from build123d import *

# Parameters (mm, degrees)
SKETCH2_OUTSIDE_W  = 26.862
SKETCH2_OUTSIDE_H  = 26.862
CUT_EXTRUDE1_DEPTH = 10
CHAMFER1_SIZE      = 0.5


with BuildPart() as part:
    # Sketch1 → Revolve1 (revolve)
    with BuildSketch(Plane(origin=(0, 0, 0), x_dir=(0, 0, -1), z_dir=(1, 0, 0)), mode=Mode.PRIVATE) as revolve1_sk:
        Polygon((0, 3.45), (0, 8.205420274), (0.373676511, 9.6), (2.426323489, 9.6), (2.8, 8.205420274), (2.8, 4.7), (4.2, 4.7), (4.2, 5.4), (7.5, 5.4), (8, 4.9), (8, 3.45), align=None)
    revolve(revolve1_sk.sketch.rotate(Axis((0, 0, 0), (0, 0, -1)), 90), axis=Axis((0, 0, 0), (0, 0, -1)))

    # Sketch2 outside → Cut-Extrude1 (cut)
    with BuildSketch(Plane.XY):
        Rectangle(SKETCH2_OUTSIDE_W, SKETCH2_OUTSIDE_H)
        Polygon((9.814954576, 0), (4.907477288, 8.5), (-4.907477288, 8.5), (-9.814954576, 0), (-4.907477288, -8.5), (4.907477288, -8.5), align=None, mode=Mode.SUBTRACT)
    extrude(amount=-CUT_EXTRUDE1_DEPTH, mode=Mode.SUBTRACT)

    # Chamfer1
    chamfer1_edges = [part.edges().sort_by_distance(p)[0] for p in [
        (-3.45, 0, 0),
        (-3.45, 0, -8),
    ]]
    chamfer(chamfer1_edges, length=CHAMFER1_SIZE)


solid = part.part
CAD build for the part. Positions are in the model's coordinates, mm. A direction names the side the tool comes from. Round coordinates to 2 decimals unless told otherwise and drop trailing zeros. Write each loop counter-clockwise with the first axis right and the second up, starting at its lowest first coordinate (ties: lowest second). Pieces come first, ordered by that corner, then holes. Notation, with made-up numbers: (56.25, -5.5) -> (93.25, -5.5) arc R26 ccw to (93.25, 27.5) -> close; hole circle Ø5 at (32.5, 17). An arc over 180 degrees is marked (long way). Answer as a JSON object with one key per item and string values.
(1) Band-saw the part on B-B, the plane y = 0. List the corners of the cut face in (x, z).
Reported:
{"outline": "(-9.6, -2.43) -> (-8.21, -2.8) -> (-4.7, -2.8) -> (-4.7, -4.2) -> (-5.4, -4.2) -> (-5.4, -7.5) -> (-4.9, -8) -> (-3.95, -8) -> (-3.45, -7.5) -> (-3.45, -0.5) -> (-3.95, 0) -> (-8.21, 0) -> (-9.6, -0.37) -> close; (3.45, -7.5) -> (3.95, -8) -> (4.9, -8) -> (5.4, -7.5) -> (5.4, -4.2) -> (4.7, -4.2) -> (4.7, -2.8) -> (8.21, -2.8) -> (9.6, -2.43) -> (9.6, -0.37) -> (8.21, 0) -> (3.95, 0) -> (3.45, -0.5) -> close"}
(2) Band-saw the part on D-D, the plane z = -3.75. List the corners of the cut face in (x, y).
Reported:
{"outline": "circle Ø9.4 at (0, 0); hole circle Ø6.9 at (0, 0)"}
(3) Pin check, flat tips, straight feed: P1, Ø1.5, axis at x = -6, z = -2.5, coming from the +Y side; P2, Ø4, axis at x = 0.5, z = -6, coming from the +Y side; P3, Ø8.5, axis at x = -0.5, y = 0.5, coming from the +Z side; P4, Ø1.5, axis at y = -3.5, z = -3, coming from the +X side. Stop position of each tip, or through.
Reported:
{"P1": "stops at y = 7.9", "P2": "stops at y = 5.4", "P3": "stops at z = 0", "P4": "stops at x = 8.19"}
(4) Which spindle directions (+Z, -Z, +X, -X, +Y, -Y) get a long thin tool onto all of the face, cutting with end or side? Do faces 1 (the face through (-7.33, 4.304, -1.382)), 2 (the face through (0, -5, -4.2)). Say none if no direction does.
Reported:
{"face 1": "+Z, -Z, -X, +Y", "face 2": "none"}
(5) Band-saw the part on C-C, the plane z = -2. List the corners of the cut face in (x, y), then the cut area to 3 significant figures.
Reported:
{"outline": "(-9.59, -0.39) -> (-5.13, -8.11) arc R9.6 ccw to (-4.46, -8.5) -> (4.46, -8.5) arc R9.6 ccw to (5.13, -8.11) -> (9.59, -0.39) arc R9.6 ccw to (9.59, 0.39) -> (5.13, 8.11) arc R9.6 ccw to (4.46, 8.5) -> (-4.46, 8.5) arc R9.6 ccw to (-5.13, 8.11) -> (-9.59, 0.39) arc R9.6 ccw to start; hole circle Ø6.9 at (0, 0)", "area": "212 mm^2"}
(6) Band-saw the part on A-A, the plane x = 0. List the corners of the cut face in (y, z).
Reported:
{"outline": "(-8.5, -2.72) -> (-8.21, -2.8) -> (-4.7, -2.8) -> (-4.7, -4.2) -> (-5.4, -4.2) -> (-5.4, -7.5) -> (-4.9, -8) -> (-3.95, -8) -> (-3.45, -7.5) -> (-3.45, -0.5) -> (-3.95, 0) -> (-8.21, 0) -> (-8.5, -0.08) -> close; (3.45, -7.5) -> (3.95, -8) -> (4.9, -8) -> (5.4, -7.5) -> (5.4, -4.2) -> (4.7, -4.2) -> (4.7, -2.8) -> (8.21, -2.8) -> (8.5, -2.72) -> (8.5, -0.08) -> (8.21, 0) -> (3.95, 0) -> (3.45, -0.5) -> close"}
(7) Two-plate mould, pull along Y, no slides. Class faces 3 (the face through (-4, -2, 0)), 4 (the face through (-4.285, 3.286, -5.873)), 5 (the face through (-2.543, -2.332, -3.951)): +Y half, -Y half, draft (parallel to the pull), parting line (faces both ways), or undercut.
Reported:
{"face 3": "draft", "face 4": "parting line", "face 5": "undercut"}
(8) Probe probe 1 along Y at (x, z) = (0, -5); probe 2 along Y at (x, z) = (0, -3.25); probe 3 along Z at (x, y) = (-3.75, 4.75). List the from-to ranges inside material, lowest first. Write a range as [from, to].
Reported:
{"probe 1": "y = [-5.4, -3.45], [3.45, 5.4]", "probe 2": "y = [-4.7, -3.45], [3.45, 4.7]", "probe 3": "z = [-2.8, 0]"}
